```python
from build123d import *

# Parameters (mm, degrees)
SKETCH9_W               = 15
SKETCH9_H               = 8.35
BOSS_EXTRUDE4_DEPTH     = 76
CUT_EXTRUDE4_DEPTH      = 46
SKETCH10_R              = 2.7
CUT_EXTRUDE5_DEPTH      = 30
SKETCH12_W              = 3
SKETCH12_H              = 3
BOSS_EXTRUDE5_DEPTH     = 5
SKETCH13_W              = 2
SKETCH13_H              = 3
CUT_EXTRUDE6_DEPTH      = 1
BOSS_EXTRUDE6_DEPTH     = 3
CUT_EXTRUDE7_REACH      = 79.472
SKETCH15_W              = 3
SKETCH15_H              = 20
CUT_EXTRUDE8_REACH      = 79.472
CUT_EXTRUDE8_END_RADIUS = 2.7
SKETCH16_R              = 2.5
BOSS_EXTRUDE8_DEPTH     = 4


with BuildPart() as part:
    # Sketch9 → Boss-Extrude4 (new body)
    with BuildSketch(Plane.XY):
        with Locations((0, 4.175)):
            Rectangle(SKETCH9_W, SKETCH9_H)
    extrude(amount=BOSS_EXTRUDE4_DEPTH)

    # Sketch7 → Cut-Extrude4 (cut)
    with BuildSketch(Plane.XY):
        Polygon((-5.5, 2), (-5.5, 5.3), (-2.75, 5.3), (-2.75, 8.35), (2.75, 8.35), (2.75, 5.3), (5.5, 5.3), (5.5, 2), align=None)
    extrude(amount=CUT_EXTRUDE4_DEPTH, mode=Mode.SUBTRACT)

    # Sketch10 → Cut-Extrude5 (cut)
    with BuildSketch(Plane.XY.offset(76)):
        with Locations((0, 4.7)):
            Circle(SKETCH10_R)
    extrude(amount=-CUT_EXTRUDE5_DEPTH, mode=Mode.SUBTRACT)

    # Sketch12 → Boss-Extrude5 (add)
    with BuildSketch(Plane(origin=(7.5, 0, 0), x_dir=(0, 0, -1), z_dir=(1, 0, 0))):
        with Locations((-71.5, 3.64)):
            Rectangle(SKETCH12_W, SKETCH12_H)
    boss_extrude5 = extrude(amount=BOSS_EXTRUDE5_DEPTH)

    # Sketch13 → Cut-Extrude6 (cut)
    with BuildSketch(Plane.XY.offset(73)):
        with Locations((10, 3.64)):
            Rectangle(SKETCH13_W, SKETCH13_H)
    cut_extrude6 = extrude(amount=-CUT_EXTRUDE6_DEPTH, mode=Mode.SUBTRACT)

    # Mirror2: Boss-Extrude5 across plane
    add(boss_extrude5.mirror(Plane(origin=(0, 0, 0), x_dir=(0, 0, 1), z_dir=(1, 0, 0))))

    # Mirror4: Cut-Extrude6 across plane
    add(cut_extrude6.mirror(Plane(origin=(0, 0, 0), x_dir=(0, 0, 1), z_dir=(1, 0, 0))), mode=Mode.SUBTRACT)

    # Sketch14 → Boss-Extrude6 (add)
    with BuildSketch(Plane(origin=(0, 5.14, 0), x_dir=(1, 0, 0), z_dir=(0, 1, 0))):
        Polygon((12.5, -70), (7.5, -66), (7.5, -70), align=None)
    boss_extrude6 = extrude(amount=-BOSS_EXTRUDE6_DEPTH)

    # Mirror5: Boss-Extrude6 across plane
    add(boss_extrude6.mirror(Plane(origin=(0, 0, 0), x_dir=(0, 0, 1), z_dir=(1, 0, 0))))

    # Sketch15 → Cut-Extrude7 (cut, up to next)
    with BuildSketch(Plane(origin=(0, 8.35, 0), x_dir=(1, 0, 0), z_dir=(0, 1, 0)), mode=Mode.PRIVATE) as cut_extrude7_sk1:
        with Locations((-5, -56.5)):
            Rectangle(SKETCH15_W, SKETCH15_H)
    cut_extrude7_tool1 = extrude(cut_extrude7_sk1.sketch, amount=-CUT_EXTRUDE7_REACH, mode=Mode.PRIVATE) & part.part
    cut_extrude7 = cut_extrude7_tool1.solids().sort_by_distance((-5, 8.35, 56.5))[0]
    add(cut_extrude7, mode=Mode.SUBTRACT)

    # Mirror6: Cut-Extrude7 across plane
    add(cut_extrude7.mirror(Plane(origin=(0, 0, 0), x_dir=(0, 0, 1), z_dir=(1, 0, 0))), mode=Mode.SUBTRACT)

    # Cut-Extrude8: up to this cylinder (the profile starts outside it)
    cut_extrude8_end = Plane(origin=(0, 4.7, 69), z_dir=(0, 0, 1)) * Cylinder(CUT_EXTRUDE8_END_RADIUS, 165.344, mode=Mode.PRIVATE)
    # Sketch16 → Cut-Extrude8 (cut, up to the surface)
    with BuildSketch(Plane.XZ, mode=Mode.PRIVATE) as cut_extrude8_sk1:
        with Locations(Location((0, 69, 0), (0, 0, 270))):
            Circle(SKETCH16_R)
    cut_extrude8_tool1 = extrude(cut_extrude8_sk1.sketch, amount=-CUT_EXTRUDE8_REACH, mode=Mode.PRIVATE) - cut_extrude8_end
    add(cut_extrude8_tool1.solids().sort_by_distance((0, 0, 69))[0], mode=Mode.SUBTRACT)

    # Sketch18 → Boss-Extrude8 (add)
    with BuildSketch(Plane.XY.offset(76)):
        Polygon((-5.5, 0), (-7.5, 0), (-7.5, -9), (7.5, -9), (7.5, 0), (5.5, 0), (5.5, -7), (-5.5, -7), align=None)
    extrude(amount=-BOSS_EXTRUDE8_DEPTH)


solid = part.part
```
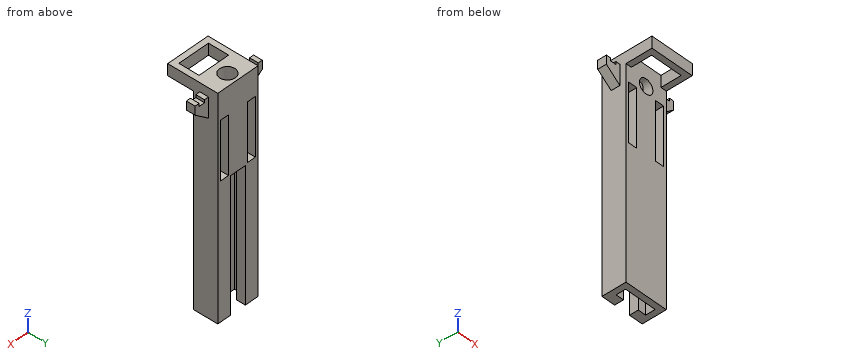
Work out the finished part from the listing and answer in its coordinate system (mm). Give positions to 0.01 mm unless a question says otherwise; leave off trailing zeros. Order: outer loops, then holes, each group sorted by start corner. A loop starts at its lowest first (then second) coordinate and runs counter-clockwise, first axis right, second up.
1. Each of these flat-tipped pins is pushed along its axis until it touches: P1, Ø6, axis at x = 0, z = 20, coming from the +Y side; P2, Ø10, axis at y = -2.5, z = 52, coming from the +X side; P3, Ø5, axis at y = -3, z = 23, coming from the +X side; P4, Ø8, axis at y = 2.5, z = 27.5, coming from the -X side. Where does it stop, or does it pass through?
Result sheet:
P1: stops at y = 8.35
P2: stops at x = 7.5
P3: passes through
P4: stops at x = -7.5
2. Section A-A, the plane y = -1.25 is taken. Determine the outline of the cut face in (x, z).
Result sheet:
outline: (-7.5, 72) - (-5.5, 72) - (-5.5, 76) - (-7.5, 76) - close; (5.5, 72) - (7.5, 72) - (7.5, 76) - (5.5, 76) - close
3. Section C-C, the plane z = 69 is taken. Determine the outline of the cut face in (x, y), and give its area (3 significant figures).
Result sheet:
outline: (-11.25, 2.14) - (-7.5, 2.14) - (-7.5, 0) - (-2.5, 0) - (-2.5, 3.68) arc R2.7 cw (long way) to (2.5, 3.68) - (2.5, 0) - (7.5, 0) - (7.5, 2.14) - (11.25, 2.14) - (11.25, 5.14) - (7.5, 5.14) - (7.5, 8.35) - (-7.5, 8.35) - (-7.5, 5.14) - (-11.25, 5.14) - close
area: 113 mm2
4. Section B-B, the plane z = 25.5 is taken. Determine the outline of the cut face in (x, y).
Result sheet:
outline: (-7.5, 0) - (7.5, 0) - (7.5, 8.35) - (2.75, 8.35) - (2.75, 5.3) - (5.5, 5.3) - (5.5, 2) - (-5.5, 2) - (-5.5, 5.3) - (-2.75, 5.3) - (-2.75, 8.35) - (-7.5, 8.35) - close
5. Straight lines are drawn through the part: L1, parallel to X at y = 4.7, z = 52; L2, parallel to Y at x = 5, z = 72.5; L3, parallel to X at y = 2, z = 69. For each, find the intervals that lie inside material, in ascending order.
Result sheet:
L1: x = -7.5 to -6.5, -3.5 to -2.7, 2.7 to 3.5, 6.5 to 7.5
L2: y = -9 to -7, 0 to 8.35
L3: x = -7.5 to -2.5, 2.5 to 7.5
